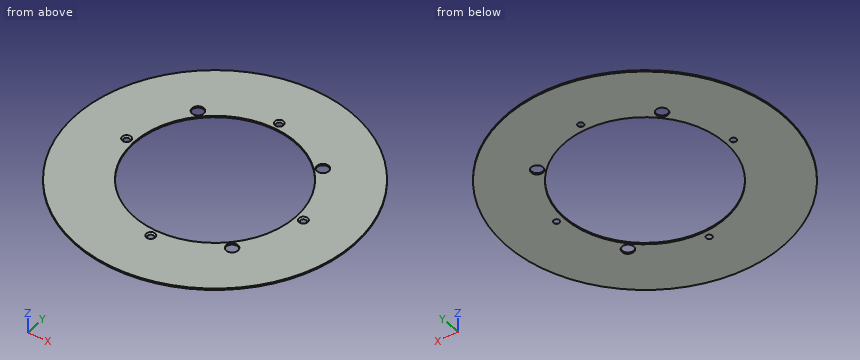
from build123d import *

# Parameters (mm, degrees)
ESQUISSE1_R                                 = 94.5
ESQUISSE1_R_2                               = 55
BOSS_EXTRU_1_DEPTH                          = 1
ENL_V_MAT_EXTRU_2_REACH                     = 135.647
ESQUISSE2_R                                 = 4
FRAISAGE_POUR_VIS_T_TE_FRAIS_E_M31_AT_COUNT = 2
FRAISAGE_POUR_VIS_T_TE_FRAIS_E_M31_AT_PITCH = 84.852813742
FRAISAGE_POUR_VIS_T_TE_FRAIS_E_M31_2_COUNT  = 2
FRAISAGE_POUR_VIS_T_TE_FRAIS_E_M31_2_PITCH  = 120
FRAISAGE_POUR_VIS_T_TE_FRAIS_E_M31_3_COUNT  = 2
FRAISAGE_POUR_VIS_T_TE_FRAIS_E_M31_3_PITCH  = 84.852813742


with BuildPart() as part:
    # Esquisse1 → Boss.-Extru.1 (new body)
    with BuildSketch(Plane.XY):
        Circle(ESQUISSE1_R)
        Circle(ESQUISSE1_R_2, mode=Mode.SUBTRACT)
    extrude(amount=BOSS_EXTRU_1_DEPTH)

    # Esquisse2 → Enlèv. mat.-Extru.2 (cut, up to next)
    with BuildSketch(Plane.XY.offset(1), mode=Mode.PRIVATE) as enl_v_mat_extru_2_sk1:
        with Locations((42.426406871, 42.426406871)):
            Circle(ESQUISSE2_R)
    enl_v_mat_extru_2_tool1 = extrude(enl_v_mat_extru_2_sk1.sketch, amount=-ENL_V_MAT_EXTRU_2_REACH, mode=Mode.PRIVATE) & part.part
    # Esquisse2 → Enlèv. mat.-Extru.2 (cut, up to next)
    with BuildSketch(Plane.XY.offset(1), mode=Mode.PRIVATE) as enl_v_mat_extru_2_sk2:
        with Locations((-42.426406871, 42.426406871)):
            Circle(ESQUISSE2_R)
    enl_v_mat_extru_2_tool2 = extrude(enl_v_mat_extru_2_sk2.sketch, amount=-ENL_V_MAT_EXTRU_2_REACH, mode=Mode.PRIVATE) & part.part
    # Esquisse2 → Enlèv. mat.-Extru.2 (cut, up to next)
    with BuildSketch(Plane.XY.offset(1), mode=Mode.PRIVATE) as enl_v_mat_extru_2_sk3:
        with Locations((42.426406871, -42.426406871)):
            Circle(ESQUISSE2_R)
    enl_v_mat_extru_2_tool3 = extrude(enl_v_mat_extru_2_sk3.sketch, amount=-ENL_V_MAT_EXTRU_2_REACH, mode=Mode.PRIVATE) & part.part
    add(enl_v_mat_extru_2_tool1.solids().sort_by_distance((42.426407, 42.426407, 1))[0], mode=Mode.SUBTRACT)
    add(enl_v_mat_extru_2_tool2.solids().sort_by_distance((-42.426407, 42.426407, 1))[0], mode=Mode.SUBTRACT)
    add(enl_v_mat_extru_2_tool3.solids().sort_by_distance((42.426407, -42.426407, 1))[0], mode=Mode.SUBTRACT)

    # Esquisse3 → Fraisage pour vis à tête fraisée M31 (revolve, cut)
    with BuildSketch(Plane(origin=(0, 60, 1), x_dir=(0, -1, 0), z_dir=(1, 0, 0))):
        Polygon((0, 0), (0, 1), (1.6, 1), (1.6, 1.4), (3, 0), align=None)
    fraisage_pour_vis_t_te_frais_e_m31 = revolve(axis=Axis((0, 60, 7.35), (0, 0, -1)), mode=Mode.SUBTRACT)

    # Fraisage pour vis à tête fraisée M31 at: Fraisage pour vis à tête fraisée M31 ×2
    with Locations(*[Vector(0.7071067811865476, -0.7071067811865476, 0) * (i * FRAISAGE_POUR_VIS_T_TE_FRAIS_E_M31_AT_PITCH) for i in range(1, FRAISAGE_POUR_VIS_T_TE_FRAIS_E_M31_AT_COUNT)]):
        add(fraisage_pour_vis_t_te_frais_e_m31, mode=Mode.SUBTRACT)

    # Fraisage pour vis _ t_te frais_e M31 2: Fraisage pour vis à tête fraisée M31 ×2
    with Locations(*[(0, -i * FRAISAGE_POUR_VIS_T_TE_FRAIS_E_M31_2_PITCH, 0) for i in range(1, FRAISAGE_POUR_VIS_T_TE_FRAIS_E_M31_2_COUNT)]):
        add(fraisage_pour_vis_t_te_frais_e_m31, mode=Mode.SUBTRACT)

    # Fraisage pour vis _ t_te frais_e M31 3: Fraisage pour vis à tête fraisée M31 ×2
    with Locations(*[Vector(-0.7071067811865476, -0.7071067811865476, 0) * (i * FRAISAGE_POUR_VIS_T_TE_FRAIS_E_M31_3_PITCH) for i in range(1, FRAISAGE_POUR_VIS_T_TE_FRAIS_E_M31_3_COUNT)]):
        add(fraisage_pour_vis_t_te_frais_e_m31, mode=Mode.SUBTRACT)


solid = part.part
Part model, mm, in its own coordinate system. Round coordinates to 2 decimals unless told otherwise and drop trailing zeros. Write each loop counter-clockwise with the first axis right and the second up, starting at its lowest first coordinate (ties: lowest second). Pieces come first, ordered by that corner, then holes. Notation, with made-up numbers: (60, -31) - (65, -31) arc R35 cw to (65, 2) - close; hole circle Ø7 at (82.5, -26). An arc over 180 degrees is marked (long way). Use CSV: the item, a comma, the result in double quotes.
Item 1: Slice it at D-D, the plane z = 0.5. Count the separate pieces of the cut face and the enclosed holes in it, then the cut area to 3 significant figures.
Results list:
separate pieces,"1"
enclosed holes,"8"
area,"18,300 mm²"
Item 2: Slice it at B-B, the plane y = 32. Write the cut outline in (x, z), then the cut area to 3 significant figures.
Results list:
outline,"(-88.92, 0) - (-44.73, 0) - (-44.73, 1) - (-88.92, 1) - close; (44.73, 0) - (88.92, 0) - (88.92, 1) - (44.73, 1) - close"
area,"88.4 mm²"
Item 3: Slice it at A-A, the plane x = 0. Write the cut outline in (y, z), then the cut area to 3 significant figures.
Results list:
outline,"(-94.5, 0) - (-62, 0) - (-63, 1) - (-94.5, 1) - close; (-58, 0) - (-55, 0) - (-55, 1) - (-57, 1) - close; (55, 0) - (58, 0) - (57, 1) - (55, 1) - close; (62, 0) - (94.5, 0) - (94.5, 1) - (63, 1) - close"
area,"69.0 mm²"
Item 4: Wall check: L1, parallel to Y at x = 0, z = 0.4; L2, parallel to X at y = -1.5, z = 0.4; L3, parallel to Y at x = 0, z = 0.6. Give the ranges that are in metal, low to high.
Results list:
L1,"y = -94.5 to -62.4, -57.6 to -55, 55 to 57.6, 62.4 to 94.5"
L2,"x = -94.49 to -61.87, -58.13 to -54.98, 54.98 to 58.13, 61.87 to 94.49"
L3,"y = -94.5 to -62.6, -57.4 to -55, 55 to 57.4, 62.6 to 94.5"
Item 5: Slice it at C-C, the plane x = -60. Write the cut outline in (y, z), then the cut area to 3 significant figures.
Results list:
outline,"(-73.01, 0) - (-2, 0) - (-3, 1) - (-73.01, 1) - close; (2, 0) - (73.01, 0) - (73.01, 1) - (3, 1) - close"
area,"141 mm²"
Item 6: Flat gauge pin, fed straight in: P1, Ø7, axis at x = -42.43, y = 42.43, coming from the -Z side. Where does the tip first touch, or does it go through?
Results list:
P1,"passes through"
